Solid Edge part; units mm, degrees
sketch "Sketch1" plane through (0, 0, 0) normal (0, -1, 0) x (1, 0, 0)
  line L0 (-73.5212, 32.2326) -> (36.4788, 32.2326)
  line L1 (36.4788, 32.2326) -> (36.4788, 42.2326)
  line L2 (36.4788, 42.2326) -> (-73.5212, 42.2326)
  line L3 (-73.5212, 42.2326) -> (-73.5212, 32.2326)
  dimension "D1" = 73.5212
  dimension "D2" = 36.4788
extrude "Protrusion1" add sketch "Sketch1" against normal blind 180
hole "Hole_1" at (36.4788, 50, 37.0863) direction (-1, 0, 0) diameter 6.35 depth 20
hole "Hole1" at (36.4788, 90, 37.0863) direction (-1, 0, 0) diameter 6.35 depth 20
hole "Hole2" at (36.4788, 120, 37.0863) direction (-1, 0, 0) diameter 6.35 depth 20
hole "Hole3" at (36.4788, 10, 37.0863) direction (-1, 0, 0) diameter 6.35 depth 20
mirror "Mirror1" about plane through (-18.5212, 90, 37.2326) normal (1, 0, 0) of "Hole_1", "Hole1", "Hole2", "Hole3"
sketch "Sketch2" plane through (-18.5212, 90, 42.2326) normal (0, 0, 1) x (-1, 0, 0)
  circle A0 centre (30, 30) radius 5
  circle A1 centre (-30, -70) radius 5
  circle A2 centre (30, -70) radius 5
  circle A3 centre (-30, -20) radius 5
  circle A4 centre (30, -20) radius 5
  circle A5 centre (-30, 30) radius 5
extrude "Cutout1" cut sketch "Sketch2" against normal through all
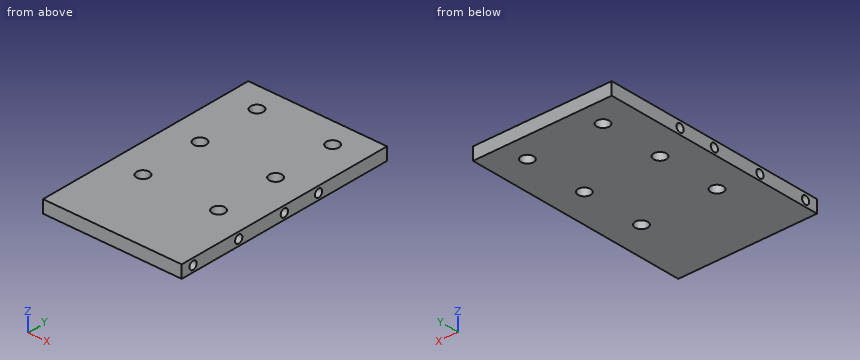
For this review, take the finished solid that the model builds, in its own axes (mm). Round coordinates to 2 decimals unless told otherwise and drop trailing zeros. Loops run counter-clockwise (first coordinate to the right, second up) from the corner with the lowest first, then second, coordinate; pieces in that order, holes last. Notation, with made-up numbers: (-10.75, 4) - (2.25, 4) arc R34 ccw to (2.25, 43) - close; hole circle Ø9 at (51, 8.25). An arc over 180 degrees is marked (long way). One line per question, with ' | ' between items.
Q1. For pin 1 (1.9 mm diameter, centred on y = 90.5, z = 36, fed in from +X); pin 2 (5.5 mm diameter, centred on y = 90, z = 37.09, fed in from -X), all flat-tipped, find the tip position at first contact; note any pin that passes through.
Taken from the geometry:
pin 1: stops at x = 16.48 | pin 2: stops at x = -53.52
Q2. Take a section at B-B (x = 27.5). Give the boundary of the cut face in (y, z) (3 decimals).
Taken from the geometry:
outline: (0, 32.233) - (180, 32.233) - (180, 42.233) - (0, 42.233) - close; hole circle Ø6.35 at (10, 37.086); hole circle Ø6.35 at (50, 37.086); hole circle Ø6.35 at (90, 37.086); hole circle Ø6.35 at (120, 37.086)
Q3. For line 1 along X through (y, z) = (60, 38.75); line 2 along Z through (x, y) = (23, 50); line 3 along X through (y, z) = (114.5, 39.75), list the stretches that pass through material, from the lowest coordinate up. Write a range as [from, to].
Taken from the geometry:
line 1: x = [-73.52, -53.52], [-43.52, 6.48], [16.48, 36.48] | line 2: z = [32.23, 33.91], [40.26, 42.23] | line 3: x = [-73.52, -50.7], [-46.34, 9.3], [13.66, 36.48]
Q4. Take a section at A-A (x = -46). Give the boundary of the cut face in (y, z).
Taken from the geometry:
outline: (0, 32.23) - (55.68, 32.23) - (55.68, 42.23) - (0, 42.23) - close; (64.32, 32.23) - (105.68, 32.23) - (105.68, 42.23) - (64.32, 42.23) - close; (114.32, 32.23) - (155.68, 32.23) - (155.68, 42.23) - (114.32, 42.23) - close; (164.32, 32.23) - (180, 32.23) - (180, 42.23) - (164.32, 42.23) - close
Q5. Take a section at D-D (x = 11.5). Give the boundary of the cut face in (y, z), and give its area (3 significant figures).
Taken from the geometry:
outline: (0, 32.23) - (55, 32.23) - (55, 42.23) - (0, 42.23) - close; (65, 32.23) - (105, 32.23) - (105, 42.23) - (65, 42.23) - close; (115, 32.23) - (155, 32.23) - (155, 42.23) - (115, 42.23) - close; (165, 32.23) - (180, 32.23) - (180, 42.23) - (165, 42.23) - close | area: 1,500 mm²
Q6. Take a section at C-C (y = 10). Give the boundary of the cut face in (x, z), and give its area (3 significant figures).
Taken from the geometry:
outline: (-73.52, 32.23) - (36.48, 32.23) - (36.48, 33.91) - (16.48, 33.91) - (16.48, 40.26) - (36.48, 40.26) - (36.48, 42.23) - (-73.52, 42.23) - (-73.52, 40.26) - (-53.52, 40.26) - (-53.52, 33.91) - (-73.52, 33.91) - close | area: 846 mm²
